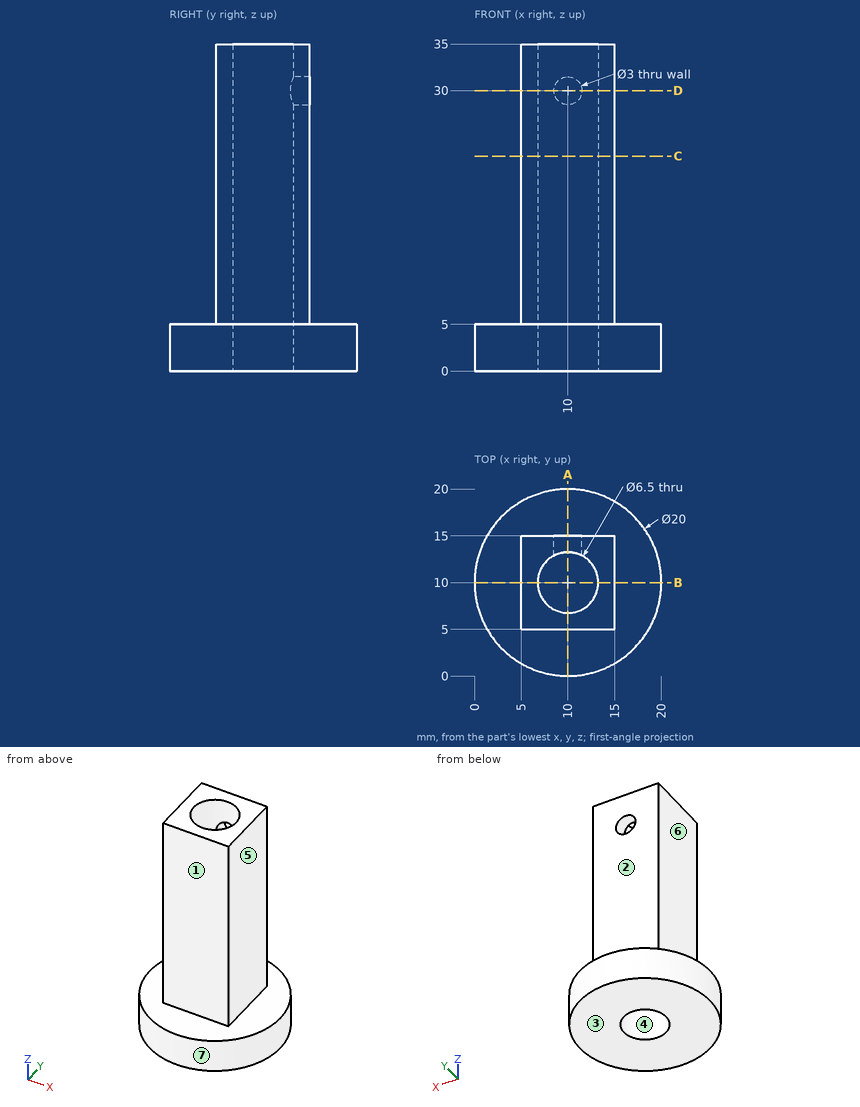
Source: three-view drawing plus pictorial views. Frame: mm from the lowest corner of the part. A direction names the side the tool comes from. Give positions to 0.01 mm unless a question says otherwise; leave off trailing zeros. Order: outer loops, then holes, each group sorted by start corner. A loop starts at its lowest first (then second) coordinate and runs counter-clockwise, first axis right, second up. Notation, with made-up numbers: (-33, 38) -> (-25, 38) arc R25 ccw to (-25, 72) -> close; hole circle Ø4 at (33, 20.5). An arc over 180 degrees is marked (long way). Use a Markdown table: item, result.
Q1. Section B-B (y = 10). Return the cut outline in (x, z), and give its area (4 significant figures).
A:
| item | result |
|---|---|
| outline | (0, 0) -> (6.75, 0) -> (6.75, 35) -> (5, 35) -> (5, 5) -> (0, 5) -> close; (13.25, 0) -> (20, 0) -> (20, 5) -> (15, 5) -> (15, 35) -> (13.25, 35) -> close |
| area | 172.5 mm^2 |
Q2. Section D-D (z = 30). Return the cut outline in (x, y), and give its area (3 significant figures).
A:
| item | result |
|---|---|
| outline | (5, 5) -> (15, 5) -> (15, 15) -> (11.5, 15) -> (11.5, 12.88) arc R3.25 cw (long way) to (8.5, 12.88) -> (8.5, 15) -> (5, 15) -> close |
| area | 61.2 mm^2 |
Q3. Pull-direction query (Y, two-part tool) for the marked faces 1, 2, 3 and 4; classes: +Y half, -Y half, draft (parallel to the pull), parting line (faces both ways), or undercut.
A:
| item | result |
|---|---|
| face 1 | -Y half |
| face 2 | +Y half |
| face 3 | draft |
| face 4 | undercut |
Q4. Section A-A (x = 10). Return the cut outline in (y, z), and give its area (3 significant figures).
A:
| item | result |
|---|---|
| outline | (0, 0) -> (6.75, 0) -> (6.75, 35) -> (5, 35) -> (5, 5) -> (0, 5) -> close; (13.25, 0) -> (20, 0) -> (20, 5) -> (15, 5) -> (15, 28.5) -> (13.25, 28.5) -> close; (13.25, 31.5) -> (15, 31.5) -> (15, 35) -> (13.25, 35) -> close |
| area | 167 mm^2 |
Q5. First-contact query: P1, Ø1.8, axis at x = 10, z = 30, coming from the +Y side; P2, Ø3, axis at x = 12, z = 24, coming from the +Y side; P3, Ø2, axis at x = 14.5, z = 16.5, coming from the -Y side. Flat tips, straight axial feed; report the tip coordinate or a pass-through.
A:
| item | result |
|---|---|
| P1 | y = 6.88 |
| P2 | y = 15 |
| P3 | y = 5 |
Q6. Section C-C (z = 23). Return the cut outline in (x, y), and give its area (3 significant figures).
A:
| item | result |
|---|---|
| outline | (5, 5) -> (15, 5) -> (15, 15) -> (5, 15) -> close; hole circle Ø6.5 at (10, 10) |
| area | 66.8 mm^2 |
Q7. Material intervals for line 1 (X direction, y = 14.2, z = 30); line 2 (Y direction, x = 10, z = 25.5); line 3 (Z direction, x = 16.75, y = 10.75), sorted ascending. Write a range as [from, to].
A:
| item | result |
|---|---|
| line 1 | [5, 8.5], [11.5, 15] |
| line 2 | [5, 6.75], [13.25, 15] |
| line 3 | [0, 5] |
Q8. Access query for the marked faces 5, 6 and 7. Directions: +Z, -Z, +X, -X, +Y, -Y. A direction counts if a zero-diameter tool reaches every point of the face in a straight line with its end or side. Return the directions, or none.
A:
| item | result |
|---|---|
| face 5 | +Z, +X, +Y, -Y |
| face 6 | +Z, -X, +Y, -Y |
| face 7 | +Z, -Z |
